from build123d import *

# Parameters (mm, degrees)
SKETCH1_W           = 700
SKETCH1_H           = 400
BOSS_EXTRUDE1_DEPTH = 80
SKETCH3_R           = 27.5
CUT_EXTRUDE1_DEPTH  = 80
SKETCH3_4_R         = 27.5
CUT_EXTRUDE2_DEPTH  = 80


with BuildPart() as part:
    # Sketch1 → Boss-Extrude1 (new body)
    with BuildSketch(Plane(origin=(0, 0, 0), x_dir=(1, 0, 0), z_dir=(0, 1, 0))):
        with Locations((28.391959799, -57.537688442)):
            Rectangle(SKETCH1_W, SKETCH1_H)
    extrude(amount=BOSS_EXTRUDE1_DEPTH)

    # Sketch3 → Cut-Extrude1 (cut)
    with BuildSketch(Plane(origin=(0, 80, 0), x_dir=(1, 0, 0), z_dir=(0, 1, 0))):
        with Locations(Location((-233.57645152, 72.474774931, 0), (0, 0, 270))):
            Circle(SKETCH3_R)
    extrude(amount=-CUT_EXTRUDE1_DEPTH, mode=Mode.SUBTRACT)

    # Sketch3_4 → Cut-Extrude2 (cut)
    with BuildSketch(Plane(origin=(0, 80, 0), x_dir=(1, 0, 0), z_dir=(0, 1, 0))):
        with Locations(Location((290.360371117, 72.474774931, 0), (0, 0, 90))):
            Circle(SKETCH3_4_R)
    extrude(amount=-CUT_EXTRUDE2_DEPTH, mode=Mode.SUBTRACT)


solid = part.part
Could you check a few things on this model? Use its own coordinates, in mm. Give positions to 0.01 mm unless a question says otherwise; leave off trailing zeros. Order: outer loops, then holes, each group sorted by start corner. A loop starts at its lowest first (then second) coordinate and runs counter-clockwise, first axis right, second up. Notation, with made-up numbers: M 6,3 L 47,3 A14 cw 47,26 Z; hole C 30.5,-4 d5. An arc over 180 degrees is marked long. One line per question, with ' | ' between items.
1. I want a section at D-D (x = 309). List the corners of the cut face in (y, z) for me, and give its area (3 significant figures).
Results:
outline: M 0,-142.46 L 80,-142.46 L 80,-92.69 L 0,-92.69 Z; M 0,-52.26 L 80,-52.26 L 80,257.54 L 0,257.54 Z | area: 28,800 mm²
2. I want a section at A-A (x = -254.5). List the corners of the cut face in (y, z) for me, and give its area (3 significant figures).
Results:
outline: M 0,-142.46 L 80,-142.46 L 80,-90.32 L 0,-90.32 Z; M 0,-54.63 L 80,-54.63 L 80,257.54 L 0,257.54 Z | area: 29,100 mm²
3. We'd pull the mould along Z, two halves only. Please class faces 1 (the face through (23, 39, -142.462)), 2 (the face through (317.206, 40.56, -66.513)), 3 (the face through (-321.608, 39, 60)): +Z half, -Z half, draft (parallel to the pull), parting line (faces both ways), or undercut.
Results:
face 1: -Z half | face 2: undercut | face 3: draft
4. I want a section at C-C (y = 47). List the corners of the cut face in (x, z) for me.
Results:
outline: M -321.61,-142.46 L 378.39,-142.46 L 378.39,257.54 L -321.61,257.54 Z; hole C -233.58,-72.47 d55; hole C 290.36,-72.47 d55
5. If I drill on line 1 (X direction, y = 60, z = -54); line 2 (X direction, y = 64.5, z = -54.5); line 3 (Z direction, x = -257, y = 76), over which ranges is the centre line in solid material (lowest first)?
Results:
line 1: -321.61 to -253.95, -213.21 to 269.99, 310.73 to 378.39 | line 2: -321.61 to -254.39, -212.76 to 269.55, 311.17 to 378.39 | line 3: -142.46 to -86.88, -58.07 to 257.54
6. I want a section at B-B (z = -86). List the corners of the cut face in (x, y) for me, and give its area (3 significant figures).
Results:
outline: M -321.61,0 L -257.52,0 L -257.52,80 L -321.61,80 Z; M -209.63,0 L 266.42,0 L 266.42,80 L -209.63,80 Z; M 314.3,0 L 378.39,0 L 378.39,80 L 314.3,80 Z | area: 48,300 mm²
